Source: CAD feature listing. Evaluate the final solid. Frame: model axes, mm. A direction names the side the tool comes from. Give positions to 0.01 mm unless a question says otherwise; leave off trailing zeros. Loops run counter-clockwise (first coordinate to the right, second up) from the corner with the lowest first, then second, coordinate; pieces in that order, holes last. Notation, with made-up numbers: (22.5, 20.5) -> (53.5, 20.5) arc R31 ccw to (53.5, 59.5) -> close; hole circle Ø6 at (68, 5). An arc over 180 degrees is marked (long way). Answer as a JSON object with one key per item and string values. Group by question number.
from build123d import *

# Parameters (mm, degrees)
F0_R     = 16
F1_DEPTH = 15
F0_R_2   = 12.5
F2_DEPTH = 1.25
F3_W     = 17
F3_H     = 12.5
F4_DEPTH = 10
F5_R     = 1.5


with BuildPart() as f1:
    # F0 (on Front) → F1 (new body)
    with BuildSketch(Plane.XZ):
        with BuildLine():
            Line((0, 25), (0, 0))
            Line((0, 0), (19.5, 0))
            Line((19.5, 0), (19.5, 3))
            Line((19.5, 3), (27, 3))
            ThreePointArc((27, 3), (43.0721423298, 9.5576629129), (51, 25))
            Line((51, 25), (51, 27.0383693291))
            ThreePointArc((51, 27.0383693291), (43.6843051192, 43.7109906775), (27, 51))
            Line((27, 51), (25.037037037, 51))
            ThreePointArc((25.037037037, 51), (7.2768537045, 43.0475290801), (0, 25))
        make_face()
        with Locations((27, 25)):
            Circle(F0_R, mode=Mode.SUBTRACT)
        with BuildLine():
            ThreePointArc((27, 51), (26.0185185185, 51.0185185185), (25.037037037, 51))
            Line((25.037037037, 51), (27, 51))
        make_face()
        with BuildLine():
            Line((51, 27.0383693291), (51, 25))
            ThreePointArc((51, 25), (51.0207833866, 26.0191846645), (51, 27.0383693291))
        make_face()
    extrude(amount=F1_DEPTH)



with BuildPart() as f1b:
    # F0 (on Front) → F1, piece 2 (new body)
    with BuildSketch(Plane.XZ):
        with Locations((27, 25)):
            Circle(F0_R_2)
    extrude(amount=F1_DEPTH)


with BuildPart() as f1_1:
    add(f1.part)

    add(f1b.part)  # F2 merges F1b
    # F0 (on Front) → F2 (join)
    with BuildSketch(Plane.XZ):
        with Locations((27, 25)):
            Circle(F0_R)
        with Locations((27, 25)):
            Circle(F0_R_2, mode=Mode.SUBTRACT)
    extrude(amount=F2_DEPTH)

    # F3 (on face) → F4 (cut)
    with BuildSketch(Plane(origin=(0, 0, 0), x_dir=(1, 0, 0), z_dir=(0, 0, -1))):
        with Locations((9.75, 7.5)):
            Rectangle(F3_W, F3_H)
    extrude(amount=-F4_DEPTH, mode=Mode.SUBTRACT)

    # F5
    f5_edges = [f1_1.edges().sort_by_distance(p)[0] for p in [
        (14.5, -15, 25),
    ]]
    fillet(f5_edges, radius=F5_R)


solid = f1_1.part
(1) Section query A-A on y = -9.75. Return the cut outline in (x, z), plus the area to 3 significant figures.
(2) Access query for faces 5 (the face through (10, -1.25, 5)), 6 (the face through (17, -1.25, 17)), 7 (the face through (0, -7, 13)), 8 (the face through (23, -7, 3)), 9 (the face through (25, 0, 26)). Directions: +Z, -Z, +X, -X, +Y, -Y. A direction counts if a zero-diameter tool reaches every point of the face in a straight line with its end or side. Return the directions, or none.
(3) Mould query, pull axis Z, two halves, no side actions, for faces 1 (the face through (17.08, -7.289, 17.394)), 2 (the face through (27, -15, 25)), 3 (the face through (23.53, -8.03, 9.38)), 4 (the face through (10, -1, 0)). Classes: pulls with the +Z half, pulls with the -Z half, needs draft (parallel to the pull), parting line crosses it, or undercut.
(4) Section query B-B on x = 8.5. Return the cut outline in (y, z), plus the area to 3 significant figures.
(5) Material intervals for line 1 (Z direction, x = 27, y = -9); line 2 (X direction, y = -2.25, z = 25.5); line 3 (X direction, y = -5, z = 15), sorted ascending. Write a range as from..to.
(6) First-contact query: pin 1 (5 mm diameter, centred on x = 13.5, z = 4, fed in from +Y); pin 2 (3 mm diameter, centred on y = -10.5, z = 6.5, fed in from +X); pin 3 (3 mm diameter, centred on x = 12.5, y = -9.5, fed in from +Z); pin 4 (6 mm diameter, centred on y = -11, z = 19.5, fed in from +X). Flat tips, straight axial feed; report the tip coordinate or a pass-through.
(7) Section query C-C on z = 39. Return the cut outline in (x, y), plus the area to 3 significant figures.
Result:
{
 "1": {"outline": "(0, 0) -> (1.25, 0) -> (1.25, 10) -> (18.25, 10) -> (18.25, 0) -> (19.5, 0) -> (19.5, 3) -> (27, 3) arc R25 ccw to (51, 25) arc R25 ccw to (27, 51) arc R26.02 ccw to (0, 25) -> close; circle Ø25 at (27, 25); hole circle Ø32 at (27, 25)", "area": "1,620 mm²"},
 "2": {"face 5": "-Z", "face 6": "-Y", "face 7": "+Z, -Z, -X, +Y, -Y", "face 8": "-Z, +X, +Y, -Y", "face 9": "+Z, -Z, +X, -X, +Y"},
 "3": {"face 1": "undercut", "face 2": "needs draft", "face 3": "undercut", "face 4": "pulls with the -Z half"},
 "4": {"outline": "(-15, 0) -> (-13.75, 0) -> (-13.75, 10) -> (-1.25, 10) -> (-1.25, 0) -> (0, 0) -> (0, 44.24) -> (-15, 44.24) -> close", "area": "539 mm²"},
 "5": {"line 1": "3..9, 12.5..37.5, 41..51", "line 2": "0..11.01, 14.51..39.49, 42.99..51.02", "line 3": "0..14.51, 19.5..34.5, 39.49..47.54"},
 "6": {"pin 1": "y = 0", "pin 2": "x = 41.2", "pin 3": "z = 48.08", "pin 4": "x = 50.57"},
 "7": {"outline": "(4.09, -15) -> (19.25, -15) -> (19.25, -1.25) -> (34.75, -1.25) -> (34.75, -15) -> (47.39, -15) -> (47.39, 0) -> (4.09, 0) -> close", "area": "436 mm²"}
}
